Geometry check sheet. Reference: drawing and pictorial views, mm from the part's lowest x, y, z. A direction names the side the tool comes from. Round coordinates to 2 decimals unless told otherwise and drop trailing zeros. Loops run counter-clockwise (first coordinate to the right, second up) from the corner with the lowest first, then second, coordinate; pieces in that order, holes last. Notation, with made-up numbers: (-10, -27) -> (46, -27) arc R10 ccw to (46, -13) -> close; hole circle Ø9 at (-5.5, 9.25). An arc over 180 degrees is marked (long way). Use one line per item in the form item = value.
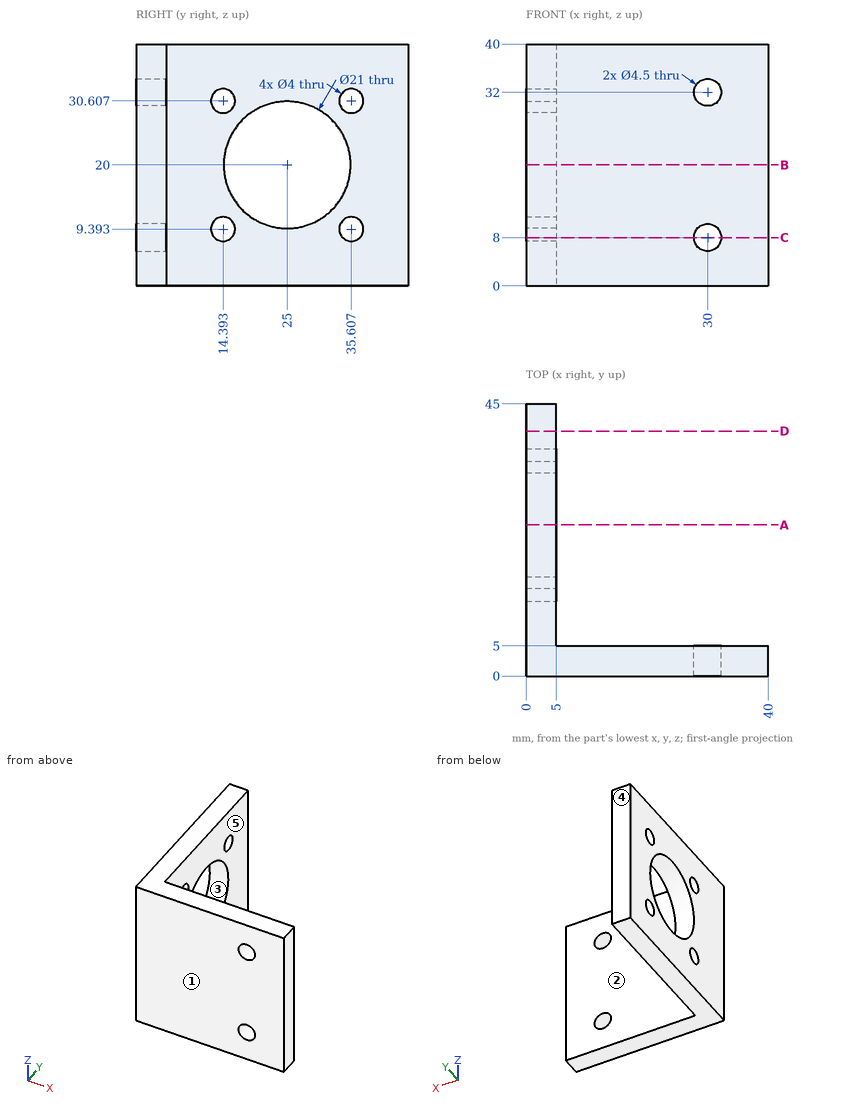
1. Tool access check on the marked faces 4 and 5. Record the directions out of +Z, -Z, +X, -X, +Y, -Y that give a thin tool (end or side, any length) a straight path to the whole face; none if there is none.
Return value:
face_4 = +Z, -Z, +X, -X, +Y
face_5 = +Z, -Z, +X, +Y
2. Section check D-D (y = 40.5). Record the boundary of the cut face in (x, z), then the cut area to 3 significant figures.
Return value:
outline = (0, 0) -> (5, 0) -> (5, 40) -> (0, 40) -> close
area = 200 mm2
3. Section check B-B (z = 20). Record the boundary of the cut face in (x, y).
Return value:
outline = (0, 0) -> (40, 0) -> (40, 5) -> (5, 5) -> (5, 14.5) -> (0, 14.5) -> close; (0, 35.5) -> (5, 35.5) -> (5, 45) -> (0, 45) -> close
4. Material ranges on line 1 along X through (y, z) = (4, 8); line 2 along Z through (x, y) = (2, 25.5); line 3 along X through (y, z) = (16, 26), recorded low to high.
Return value:
line_1 = 0 to 27.75, 32.25 to 40
line_2 = 0 to 9.51, 30.49 to 40
line_3 = 0 to 5
5. Section check A-A (y = 25). Record the boundary of the cut face in (x, z).
Return value:
outline = (0, 0) -> (5, 0) -> (5, 9.5) -> (0, 9.5) -> close; (0, 30.5) -> (5, 30.5) -> (5, 40) -> (0, 40) -> close
6. Gauge pin test, flat ends, axial feed: pin 1 (12 mm diameter, centred on y = 29, z = 10.5, fed in from +X); pin 2 (2.5 mm diameter, centred on y = 35.61, z = 30.61, fed in from +X); pin 3 (10 mm diameter, centred on x = 31.5, z = 31, fed in from +Y). Record the tip position at first contact, or that the pin passes through.
Return value:
pin_1 = 5
pin_2 = through
pin_3 = 5
7. Section check C-C (z = 8). Record the boundary of the cut face in (x, y), then the cut area to 3 significant figures.
Return value:
outline = (0, 0) -> (27.75, 0) -> (27.75, 5) -> (5, 5) -> (5, 12.96) -> (0, 12.96) -> close; (0, 15.83) -> (5, 15.83) -> (5, 34.17) -> (0, 34.17) -> close; (0, 37.04) -> (5, 37.04) -> (5, 45) -> (0, 45) -> close; (32.25, 0) -> (40, 0) -> (40, 5) -> (32.25, 5) -> close
area = 349 mm2
8. Mould release check, pull along Y, two halves, no side actions. Record for the marked faces 1, 2 and 3: released by +Y, released by -Y, zero draft, split by the parting line, or undercut.
Return value:
face_1 = released by -Y
face_2 = released by +Y
face_3 = undercut
